from build123d import *

# Parameters (mm, degrees)
SKETCH1_W             = 105
SKETCH1_H             = 202
BOSS_EXTRUDE1_DEPTH   = 16
SKETCH2_W             = 95
SKETCH2_H             = 192
CUT_EXTRUDE1_DEPTH    = 11
CUT_EXTRUDE2_DEPTH    = 5
LPATTERN1_COUNT       = 7
LPATTERN1_PITCH       = 25
CUT_EXTRUDE4_DEPTH    = 287
FILLET1_R             = 6
FILLET2_R             = 1
M3_TAPPED_HOLE1_D     = 2.5
M3_TAPPED_HOLE1_DEPTH = 7.5
M3_TAPPED_HOLE1_TIP   = 0.751075774
M3_TAPPED_HOLE2_D     = 2.5
M3_TAPPED_HOLE2_DEPTH = 7.5
M3_TAPPED_HOLE2_TIP   = 0.751075774


with BuildPart() as part:
    # Sketch1 → Boss-Extrude1 (new body)
    with BuildSketch(Plane.XY):
        with Locations((52.5, 101)):
            Rectangle(SKETCH1_W, SKETCH1_H)
    extrude(amount=BOSS_EXTRUDE1_DEPTH)

    # Sketch2 → Cut-Extrude1 (cut)
    with BuildSketch(Plane.XY.offset(16)):
        with Locations((52.5, 101)):
            Rectangle(SKETCH2_W, SKETCH2_H)
    extrude(amount=-CUT_EXTRUDE1_DEPTH, mode=Mode.SUBTRACT)

    # Sketch3 → Cut-Extrude2 (cut)
    with BuildSketch(Plane.XY.offset(5)):
        with BuildLine():
            Line((17.5, 187), (87.5, 187))
            ThreePointArc((87.5, 187), (95, 179.5), (87.5, 172))
            Line((87.5, 172), (17.5, 172))
            ThreePointArc((17.5, 172), (10, 179.5), (17.5, 187))
        make_face()
    cut_extrude2 = extrude(amount=-CUT_EXTRUDE2_DEPTH, mode=Mode.SUBTRACT)

    # LPattern1: Cut-Extrude2 ×7
    with Locations(*[(0, -i * LPATTERN1_PITCH, 0) for i in range(1, LPATTERN1_COUNT)]):
        add(cut_extrude2, mode=Mode.SUBTRACT)

    # Sketch5 → Cut-Extrude4 (cut)
    with BuildSketch(Plane.XZ):
        with BuildLine():
            Line((17.5, 7), (17.5, 9))
            ThreePointArc((17.5, 9), (18.085786438, 10.414213562), (19.5, 11))
            Line((19.5, 11), (35.5, 11))
            ThreePointArc((35.5, 11), (36.914213562, 10.414213562), (37.5, 9))
            Line((37.5, 9), (37.5, 7))
            ThreePointArc((37.5, 7), (36.914213562, 5.585786438), (35.5, 5))
            Line((35.5, 5), (19.5, 5))
            ThreePointArc((19.5, 5), (18.085786438, 5.585786438), (17.5, 7))
        make_face()
        with BuildLine():
            Line((87.5, 9), (87.5, 7))
            ThreePointArc((87.5, 7), (86.914213562, 5.585786438), (85.5, 5))
            Line((85.5, 5), (69.5, 5))
            ThreePointArc((69.5, 5), (68.085786438, 5.585786438), (67.5, 7))
            Line((67.5, 7), (67.5, 9))
            ThreePointArc((67.5, 9), (68.085786438, 10.414213562), (69.5, 11))
            Line((69.5, 11), (85.5, 11))
            ThreePointArc((85.5, 11), (86.914213562, 10.414213562), (87.5, 9))
        make_face()
    extrude(amount=-CUT_EXTRUDE4_DEPTH, mode=Mode.SUBTRACT)

    # Fillet1
    fillet1_edges = [part.edges().sort_by_distance(p)[0] for p in [
        (0, 202, 8),
        (105, 202, 8),
        (105, 0, 8),
        (0, 0, 8),
    ]]
    fillet(fillet1_edges, radius=FILLET1_R)

    # Fillet2
    fillet2_edges = [part.edges().sort_by_distance(p)[0] for p in [
        (100, 197, 10.5),
        (5, 197, 10.5),
        (5, 5, 10.5),
        (100, 5, 10.5),
    ]]
    fillet(fillet2_edges, radius=FILLET2_R)

    # M3 Tapped Hole1
    with Locations(Plane(origin=(92.5, 202, 8), x_dir=(0, 0, 1), z_dir=(0, 1, 0))):
        with Locations((0, 0), (0, -40), (0, -80)):
            Hole(M3_TAPPED_HOLE1_D / 2, depth=M3_TAPPED_HOLE1_DEPTH)
            with Locations((0, 0, -(M3_TAPPED_HOLE1_DEPTH + M3_TAPPED_HOLE1_TIP / 2))):  # 118° drill point
                Cone(0, M3_TAPPED_HOLE1_D / 2, M3_TAPPED_HOLE1_TIP, mode=Mode.SUBTRACT)

    # M3 Tapped Hole2
    with Locations(Plane(origin=(12.5, 0, 8), x_dir=(0, 0, -1), z_dir=(0, -1, 0))):
        with Locations((0, 0), (0, 40), (0, 80)):
            Hole(M3_TAPPED_HOLE2_D / 2, depth=M3_TAPPED_HOLE2_DEPTH)
            with Locations((0, 0, -(M3_TAPPED_HOLE2_DEPTH + M3_TAPPED_HOLE2_TIP / 2))):  # 118° drill point
                Cone(0, M3_TAPPED_HOLE2_D / 2, M3_TAPPED_HOLE2_TIP, mode=Mode.SUBTRACT)


solid = part.part
Part model, mm, in its own coordinate system. A direction names the side the tool comes from. Give positions to 0.01 mm unless a question says otherwise; leave off trailing zeros. Loops run counter-clockwise (first coordinate to the right, second up) from the corner with the lowest first, then second, coordinate; pieces in that order, holes last.
(1) Band-saw the part on C-C (x = 60). Count the separate pieces of the cut face and the enclosed holes in it, and give its area (3 significant figures).
Return value:
separate pieces: 8
enclosed holes: 0
area: 595 mm2
(2) Band-saw the part on A-A (y = 154.5). Write the cut outline in (x, z).
Return value:
outline: (0, 0) - (10, 0) - (10, 5) - (5, 5) - (5, 16) - (0, 16) - close; (95, 0) - (105, 0) - (105, 16) - (100, 16) - (100, 5) - (95, 5) - close
(3) 3-axis set-ups, long thin cutter, end or side, ignore diameter. For faces 1 (the flat face through (52, 87, 3)), 2 (the flat face through (52, 197, 12)), 3 (the flat face through (77, 199, 11)), 4 (the cylindrical face through (103.289, 1.804, 8.112)): which of +Z, -Z, +X, -X, +Y, -Y reach the whole face in a straight line?
Return value:
face 1: +Z, -Z
face 2: +Z
face 3: +Y, -Y
face 4: +Z, -Z, +X, -Y
(4) Pin check, flat tips, straight feed: pin 1 (5 mm diameter, centred on x = 15.5, y = 165, fed in from +Z); pin 2 (1.6 mm diameter, centred on y = 199.5, z = 8, fed in from +X); pin 3 (1.6 mm diameter, centred on y = 199.5, z = 8.5, fed in from -X). Stop position of each tip, or through.
Return value:
pin 1: stops at z = 5
pin 2: stops at x = 104.36
pin 3: stops at x = 0.64
(5) Drill centre lines: line 1 along Z through (x, y) = (92.5, 200.75); line 2 along Y through (x, z) = (16.5, 13.25); line 3 along X through (y, z) = (198.9, 8). Where is each one in solid material? Low to high.
Return value:
line 1: z = 0 to 6.75, 9.25 to 16
line 2: y = 0 to 5, 197 to 202
line 3: x = 0.75 to 11.25, 13.75 to 17.5, 37.5 to 51.25, 53.75 to 67.5, 87.5 to 91.25, 93.75 to 104.25
(6) Band-saw the part on B-B (z = 13.25). Write the cut outline in (x, y), and give its area (3 significant figures).
Return value:
outline: (0, 6) arc R6 ccw to (6, 0) - (99, 0) arc R6 ccw to (105, 6) - (105, 196) arc R6 ccw to (99, 202) - (6, 202) arc R6 ccw to (0, 196) - close; hole (5, 6) arc R1 ccw to (6, 5) - (99, 5) arc R1 ccw to (100, 6) - (100, 196) arc R1 ccw to (99, 197) - (6, 197) arc R1 ccw to (5, 196) - close
area: 2,940 mm2
(7) Pull direction Z, two halves, no side cores. Call faces 5 (the flat face through (2, 101, 16)), 6 (the flat face through (27, 2, 11)), 7 (the flat face through (105, 100, 8)): pulls with the +Z half, pulls with the -Z half, needs draft (parallel to the pull), parting line crosses it, or undercut.
Return value:
face 5: pulls with the +Z half
face 6: undercut
face 7: needs draft
